Autodesk Inventor part; units mm, degrees
ref_plane "Work Plane2" through (-100, 0, 190) normal (0, 0, 1) x (1, 0, 0)
ref_plane "YZ Plane" through (0, 0, 0) normal (1, 0, 0) x (0, 1, 0)
ref_plane "XZ Plane" through (0, 0, 0) normal (0, 1, 0) x (-1, 0, 0)
sketch "Sketch1" plane through (0, 0, 0) normal (0, 1, 0) x (-1, 0, 0)
  line L0 (-200, 300) -> (200, 300)
  line L1 (200, 300) -> (200, -300)
  line L2 (200, -300) -> (-200, -300)
  line L3 (-200, -300) -> (-200, 300)
  line L4 (-200, 300) -> (200, -300) construction
  line L5 (200, 300) -> (-200, -300) construction
  point P0 (0, 0)
  dimension "d0" = 400
  dimension "d1" = 600
extrude "Extrusion1" add sketch "Sketch1" along normal blind 2
sketch "Sketch2" plane through (0, 2, 0) normal (0, 1, 0) x (1, 0, 0)
  line L0 (200, 300) -> (-200, 300)
  line L1 (-200, 300) -> (-200, 275)
  line L2 (-200, 300) -> (-200, -300)
  line L3 (-200, 300) -> (-100, 300)
  line L4 (-100, 300) -> (-200, 275)
  line L5 (-200, 275) -> (-200, 250)
  line L6 (-200, 250) -> (-175, 250)
  line L7 (-175, 250) -> (-175, 150)
  line L8 (-175, 150) -> (-200, 150)
  line L9 (-200, 250) -> (-200, 150)
  line L10 (0, 250) -> (0, 74.4907)
  line L11 (-155.9773, 0) -> (157.8952, 0)
  line L12 (-200, 300) -> (200, 300)
  line L13 (200, 300) -> (200, -300)
  line L14 (100, 300) -> (200, 275)
  line L15 (200, 250) -> (175, 250)
  line L16 (175, 250) -> (175, 150)
  line L17 (175, 150) -> (200, 150)
  line L18 (200, -300) -> (-200, -300)
  line L19 (-200, -300) -> (-200, -275)
  line L20 (-200, -300) -> (-100, -300)
  line L21 (-100, -300) -> (-200, -275)
  line L22 (-200, -275) -> (-200, -250)
  line L23 (-200, -250) -> (-200, -150)
  line L24 (200, -300) -> (200, 300)
  line L25 (100, -300) -> (200, -275)
  line L26 (-200, -300) -> (200, -300)
  point P0 (0, 0)
  dimension "d4" = 25
  dimension "d5" = 100
  dimension "d6" = 25
  dimension "d7" = 25
  dimension "d8" = 100
extrude "Extrusion2" cut sketch "Sketch2" against normal blind 2 contours L13 L14 L0 | L4 L1 L0 | L13 L17 L16 L15 | L6 L7 L8 L2 | L13 L18 L25 | L18 L2 L21
mirror "Mirror2" about plane through (0, 0, 0) normal (1, 0, 0)
ref_plane "Work Plane2" through (-100, 0, 190) normal (0, 0, 1) x (1, 0, 0)
mirror "Mirror4" about plane through (-100, 0, 190) normal (0, 0, 1) of "Mirror2"
sketch "Sketch13" plane through (0, 2, 0) normal (0, 1, 0) x (1, 0, 0)
  line L0 (-200, 150) -> (-200, -275)
  line L1 (-200, 0) -> (-200, 150)
  line L2 (-200, 150) -> (200, 150)
  line L3 (200, 150) -> (200, -150)
  line L4 (200, -150) -> (-200, -150)
  line L5 (-200, 0) -> (-200, 50)
  line L6 (-200, 50) -> (200, 50)
  line L7 (-200, 50) -> (-200, 595.1707)
  line L8 (-200, 595.1707) -> (291.7949, 595.1707)
  line L9 (291.7949, 595.1707) -> (291.7949, 150)
  line L10 (291.7949, 150) -> (200, 150)
  line L11 (-200, -150) -> (-200, -431.5542)
  line L12 (-200, -431.5542) -> (200, -431.5542)
  line L13 (200, -431.5542) -> (200, -150)
  point P0 (0, 0)
  dimension "d71" = 400
  dimension "d72" = 300
  dimension "d73" = 50
extrude "Extrusion11" cut sketch "Sketch13" against normal blind 10 contours L2 L3 L6 L0 | L7 L8 L9 L10 L2 | L4 L13 L12 L11 L0
sketch "Sketch14" plane through (0, 2, 0) normal (0, 1, 0) x (1, 0, 0)
  line L0 (-250, 100) -> (-150, 100)
  line L1 (-150, 100) -> (-150, 0)
  line L2 (-150, 0) -> (-250, 0)
  line L3 (-250, 0) -> (-250, 100)
  line L4 (-200, 50) -> (-200, -150)
  line L5 (-250, 100) -> (-150, 0) construction
  line L6 (-150, 100) -> (-250, 0) construction
  line L7 (200, 50) -> (-200, 50)
  line L8 (-150, 50) -> (-200, 0)
  line L9 (-200, 50) -> (-200, -50)
  line L10 (-200, -50) -> (200, -50)
  line L11 (0, 0) -> (0, -87.9853)
  line L12 (-250, -200) -> (-150, -200)
  line L13 (-150, -200) -> (-150, -100)
  line L14 (-150, -100) -> (-250, -100)
  line L15 (-250, -100) -> (-250, -200)
  line L16 (-150, -150) -> (-200, -100)
  line L17 (250, 100) -> (150, 100)
  line L18 (150, 100) -> (150, 0)
  line L19 (150, 0) -> (250, 0)
  line L20 (250, 0) -> (250, 100)
  line L21 (150, 50) -> (200, 0)
  line L22 (250, -200) -> (150, -200)
  line L23 (250, -100) -> (250, -200)
  line L24 (150, -100) -> (250, -100)
  line L25 (150, -150) -> (200, -100)
  line L26 (150, -200) -> (150, -100)
  dimension "d76" = 100
  dimension "d77" = 100
  dimension "d78" = 100
extrude "Extrusion12" cut sketch "Sketch14" against normal blind 10 contours L0 L1 L7 L4 L2 L3 | L8 L4 L7 | L15 L14 L16 L13 L12 | L20 L19 L21 L18 L17 | L22 L26 L25 L24 L23
sketch "Sketch15" plane through (0, 2, 0) normal (0, 1, 0) x (1, 0, 0)
  line L0 (-200, 0) -> (-200, -100)
  line L1 (-200, 0) -> (-200, -30)
  line L2 (-200, -30) -> (-170, -30)
  line L3 (-170, -30) -> (-170, 0)
  line L4 (-180, -15) -> (-180, -16)
  line L5 (-180, -16) -> (-180, -15)
  line L6 (-180, -15) -> (-180, -14)
  circle A0 centre (-180, -7.5) radius 4
  circle A1 centre (-180, -22.5) radius 4
  line L7 (0, 0) -> (0, -46.3113)
  circle A2 centre (180, -7.5) radius 4
  circle A3 centre (180, -22.5) radius 4
  dimension "d81" = 30
  dimension "d82" = 30
  dimension "d86" = 1
  dimension "d89" = 8
  dimension "d99" = 15
extrude "Extrusion13" cut sketch "Sketch15" against normal blind 10
sketch "Sketch16" plane through (0, 2, 0) normal (0, 1, 0) x (1, 0, 0)
  circle A0 centre (-80, -99.9978) radius 4
  circle A1 centre (70, -99.9978) radius 4
  circle A2 centre (7.5, -92.5769) radius 4
  circle A3 centre (-7.5, -92.5769) radius 4
  line L0 (0, -99.9978) -> (0, -89.9978)
  line L1 (0, -99.9978) -> (0, -91.9978)
  point P0 (0, 0)
  dimension "d95" = 8
  dimension "d96" = 8
  dimension "d106" = 8
extrude "Extrusion14" cut sketch "Sketch16" against normal blind 10 contours A2 | A3
ref_plane "Work Plane1" through (0, 0, 0) normal (1, 0, 0) x (0, 1, 0)
ref_plane "Work Plane3" through (0, 0, 380) normal (-1, 0, 0) x (0, 1, 0)
ref_plane "Work Plane4" through (0, 0, 380) normal (-1, 0, 0) x (0, 1, 0)
properties part number "chassis up" material "Steel, Mild"
Verification items for the finished model (mm, model axes). Coordinates: 2 decimals unless noted, no trailing zeros. Loops run counter-clockwise (first coordinate to the right, second up) from the corner with the lowest first, then second, coordinate; pieces in that order, holes last. Notation, with made-up numbers: (-10, 40.25) -> (-2, 40.25) arc R14 cw to (-2, 55.25) -> close; hole circle Ø1 at (-33.75, 16). An arc over 180 degrees is marked (long way). Answer as a JSON object with one key per item and string values. Group by question number.
Item 1: Sectioned sample at D-D on y = 1.3. Record the boundary of the cut face in (x, z), plus the area to 3 significant figures.
Item 2: Mould release check, pull along Z, two halves, no side actions. Record for faces 1 (the cylindrical face through (-176.185, 1.014, 21.299)), 2 (the flat face through (3, 2, 51)), 3 (the flat face through (-175, 1, -25)), 4 (the cylindrical face through (9.346, 1.014, 96.126)): +Z half, -Z half, draft (parallel to the pull), parting line (faces both ways), or undercut.
Item 3: Depth check by flat-ended pin: pin 1 (6.5 mm diameter, centred on x = -7.5, z = 92.58, fed in from -Y). Enter the tip coordinate at first touch or a pass-through.
Item 4: Scan lines: probe 1 along X at (y, z) = (1.5, 7.5); probe 2 along Z at (x, y) = (-180, 0.5); probe 3 along Z at (x, y) = (7.5, 1.05). Record each from-to range of solid material in increasing order.
Item 5: Sectioned sample at A-A on x = -7.5. Record the boundary of the cut face in (y, z), plus the area to 3 significant figures.
Item 6: Sectioned sample at C-C on x = 180. Record the boundary of the cut face in (y, z).
Item 7: Sectioned sample at B-B on z = 22.5. Record the boundary of the cut face in (x, y).
Evaluation:
{
 "1": {"outline": "(-200, 0) -> (-150, -50) -> (150, -50) -> (200, 0) -> (200, 100) -> (150, 150) -> (-150, 150) -> (-200, 100) -> close; hole circle Ø8 at (-180, 7.5); hole circle Ø8 at (-180, 22.5); hole circle Ø8 at (-7.5, 92.58); hole circle Ø8 at (7.5, 92.58); hole circle Ø8 at (180, 7.5); hole circle Ø8 at (180, 22.5)", "area": "74,700 mm²"},
 "2": {"face 1": "undercut", "face 2": "draft", "face 3": "-Z half", "face 4": "undercut"},
 "3": {"pin 1": "passes through"},
 "4": {"probe 1": "x = -200 to -184, -176 to 176, 184 to 200", "probe 2": "z = -20 to 3.5, 11.5 to 18.5, 26.5 to 120", "probe 3": "z = -50 to 88.58, 96.58 to 150"},
 "5": {"outline": "(0, -50) -> (2, -50) -> (2, 88.58) -> (0, 88.58) -> close; (0, 96.58) -> (2, 96.58) -> (2, 150) -> (0, 150) -> close", "area": "384 mm²"},
 "6": {"outline": "(0, -20) -> (2, -20) -> (2, 3.5) -> (0, 3.5) -> close; (0, 11.5) -> (2, 11.5) -> (2, 18.5) -> (0, 18.5) -> close; (0, 26.5) -> (2, 26.5) -> (2, 120) -> (0, 120) -> close"},
 "7": {"outline": "(-200, 0) -> (-184, 0) -> (-184, 2) -> (-200, 2) -> close; (-176, 0) -> (176, 0) -> (176, 2) -> (-176, 2) -> close; (184, 0) -> (200, 0) -> (200, 2) -> (184, 2) -> close"}
}
